Part model, mm, in its own coordinate system. Give positions to 0.01 mm unless a question says otherwise; leave off trailing zeros. Loops run counter-clockwise (first coordinate to the right, second up) from the corner with the lowest first, then second, coordinate; pieces in that order, holes last. Notation, with made-up numbers: (82.25, -8) -> (95.25, -8) arc R18 cw to (95.25, 10) -> close; hole circle Ø1 at (10.25, -23). An arc over 180 degrees is marked (long way). Write item = value, one per line.
from build123d import *

# Parameters (mm, degrees)
BOSS_EXTRUDE1_DEPTH = 500
SKETCH2_R           = 3
CUT_EXTRUDE1_DEPTH  = 501.423820376
SKETCH3_R           = 4.75
CUT_EXTRUDE2_DEPTH  = 8.5
LPATTERN1_COUNT     = 100
LPATTERN1_PITCH     = 60


with BuildPart() as part:
    # Sketch1 → Boss-Extrude1 (new body)
    with BuildSketch(Plane.XY):
        with BuildLine():
            Line((-6.55, -4.115), (-6.55, -7.045))
            Line((-6.55, -7.045), (-10, -10.495))
            Line((-10, -10.495), (-10, -13.495))
            Line((-10, -13.495), (-9, -14.495))
            Line((-9, -14.495), (0, -14.495))
            Line((0, -14.495), (0, 3.505))
            Line((0, 3.505), (-7.16, 3.505))
            Line((-7.16, 3.505), (-7.768111832, 2.896888168))
            ThreePointArc((-7.768111832, 2.896888168), (-8.334356479, 1.761574733), (-9.469669914, 1.195330086))
            Line((-9.469669914, 1.195330086), (-10, 0.665))
            Line((-10, 0.665), (-10, -0.665))
            Line((-10, -0.665), (-9.469669914, -1.195330086))
            ThreePointArc((-9.469669914, -1.195330086), (-8.334356479, -1.761574733), (-7.768111832, -2.896888168))
            Line((-7.768111832, -2.896888168), (-6.55, -4.115))
        make_face()
    boss_extrude1 = extrude(amount=BOSS_EXTRUDE1_DEPTH)

    # Mirror1: Boss-Extrude1 across plane
    add(boss_extrude1.mirror(Plane(origin=(0, 3.505, 500), x_dir=(0, 0, 1), z_dir=(-1, 0, 0))))

    # Sketch2 → Cut-Extrude1 (cut, through all)
    with BuildSketch(Plane(origin=(0, 3.505, 0), x_dir=(1, 0, 0), z_dir=(0, 1, 0))):
        with Locations(Location((0, -30, 0), (0, 0, 270))):
            Circle(SKETCH2_R)
    cut_extrude1 = extrude(amount=-CUT_EXTRUDE1_DEPTH, mode=Mode.SUBTRACT)

    # Sketch3 → Cut-Extrude2 (cut)
    with BuildSketch(Plane(origin=(0, 3.505, 0), x_dir=(1, 0, 0), z_dir=(0, 1, 0))):
        with Locations(Location((0, -30, 0), (0, 0, 270))):
            Circle(SKETCH3_R)
    cut_extrude2 = extrude(amount=-CUT_EXTRUDE2_DEPTH, mode=Mode.SUBTRACT)

    # LPattern1: Cut-Extrude1, Cut-Extrude2 ×100
    with Locations(*[(0, 0, i * LPATTERN1_PITCH) for i in range(1, LPATTERN1_COUNT)]):
        add(cut_extrude1, mode=Mode.SUBTRACT)
        add(cut_extrude2, mode=Mode.SUBTRACT)

    # Mirror2: part across plane


with BuildPart() as part_1:
    add(part.part)
    add(part.part.mirror(Plane(origin=(-9.748570041, -3.175788295, 0), x_dir=(1, 0, 0), z_dir=(0, 0, -1))))


solid = part_1.part
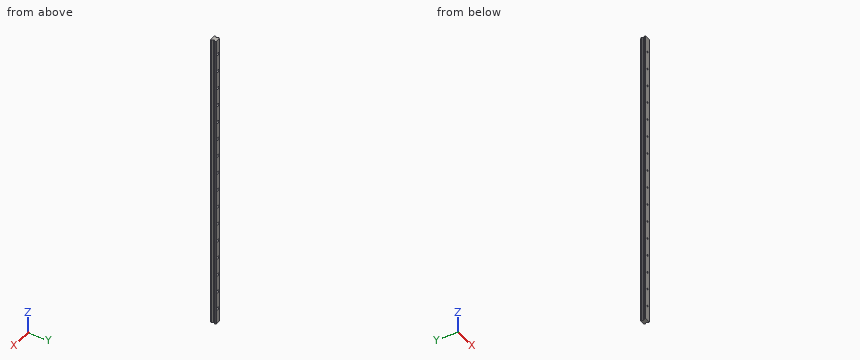
1) Slice it at B-B, the plane z = -16.5. List the corners of the cut face in (x, y) (3 decimals), and give its area (3 significant figures).
Resolved:
outline = (-10, -13.495) -> (-9, -14.495) -> (9, -14.495) -> (10, -13.495) -> (10, -10.495) -> (6.55, -7.045) -> (6.55, -4.115) -> (7.768, -2.897) arc R2 cw to (9.47, -1.195) -> (10, -0.665) -> (10, 0.665) -> (9.47, 1.195) arc R2 cw to (7.768, 2.897) -> (7.16, 3.505) -> (-7.16, 3.505) -> (-7.768, 2.897) arc R2 cw to (-9.47, 1.195) -> (-10, 0.665) -> (-10, -0.665) -> (-9.47, -1.195) arc R2 cw to (-7.768, -2.897) -> (-6.55, -4.115) -> (-6.55, -7.045) -> (-10, -10.495) -> close
area = 304 mm²
2) Drill centre lines: line 1 along X through (y, z) = (-3.5, 390) (3 decimals); line 2 along X through (y, z) = (-2.5, -210); line 3 along Y through (x, z) = (8.5, 397) (3 decimals). Where is each one in solid material? Low to high. Write a range as [from, to].
Resolved:
line_1 = [-7.165, -4.75], [4.75, 7.165]
line_2 = [-7.87, -4.75], [4.75, 7.87]
line_3 = [-14.495, -8.995], [-1.613, 1.613]
3) Drop flat-ended pins along their axis: P1, Ø2.5, axis at y = -5.5, z = 62, coming from the -X side; P2, Ø5.5, axis at x = 0, z = -30, coming from the -Y side; P3, Ø2.5, axis at y = -5, z = 9.5, coming from the +X side (3 decimals); P4, Ø8, axis at x = 0, z = -90, coming from the +Y side (3 decimals). Give the stop position or say it passes through.
Resolved:
P1 = -6.55
P2 = through
P3 = 6.915
P4 = -4.995
4) Slice it at A-A, the plane x = 0. Count the separate pieces of the cut face and the enclosed holes in it, and give its area (3 significant figures).
Resolved:
separate_pieces = 17
enclosed_holes = 0
area = 15,800 mm²
